Geometry check sheet. Reference: the model listing, model coordinates, mm. A direction names the side the tool comes from. Give positions to 0.01 mm unless a question says otherwise; leave off trailing zeros. Order: outer loops, then holes, each group sorted by start corner. A loop starts at its lowest first (then second) coordinate and runs counter-clockwise, first axis right, second up. Notation, with made-up numbers: (44, -32) - (55, -32) arc R16 cw to (55, -5) - close; hole circle Ø8 at (-2, 7). An arc over 180 degrees is marked (long way). Put each result on its own line as item: value. Start each with the question number.
```python
from build123d import *

# Parameters (mm, degrees)
F0_R     = 4
F0_R_2   = 1.5
F1_DEPTH = 20
F3_R     = 1.1
F4_DEPTH = 16.001


with BuildPart() as f1:
    # F0 (on Top) → F1 (new body)
    with BuildSketch(Plane.XY):
        with BuildLine():
            ThreePointArc((-8, 0), (0, -8), (8, 0))
            Line((8, 0), (8, 24))
            ThreePointArc((8, 24), (7.12132, 26.12132), (5, 27))
            Line((5, 27), (-5, 27))
            ThreePointArc((-5, 27), (-7.12132, 26.12132), (-8, 24))
            Line((-8, 24), (-8, 0))
        make_face()
        Circle(F0_R, mode=Mode.SUBTRACT)
        with Locations((-3.675823, 22.163428)):
            Circle(F0_R_2, mode=Mode.SUBTRACT)
        with Locations((3.675823, 22.163428)):
            Circle(F0_R_2, mode=Mode.SUBTRACT)
    extrude(amount=F1_DEPTH)

    # F3 (on face) → F4 (cut, through all)
    with BuildSketch(Plane(origin=(-8, 0, 0), x_dir=(0, -1, 0), z_dir=(-1, 0, 0))):
        with BuildLine():
            Line((15.480949, 34.118096), (-11.102321, 34.118096))
            Line((-11.102321, 34.118096), (-11.102321, 15))
            ThreePointArc((-11.102321, 15), (-9.637855, 11.464466), (-6.102321, 10))
            Line((-6.102321, 10), (15.473341, 10))
            Line((15.473341, 10), (15.480949, 34.118096))
        make_face()
        with BuildLine():
            Line((-19.958727, 15), (-48.31529, 15))
            Line((-48.31529, 15), (-48.31529, 0))
            Line((-48.31529, 0), (-48.31529, -8.176547))
            Line((-48.31529, -8.176547), (-5.153973, -8.176547))
            Line((-5.153973, -8.176547), (-5.153973, 0))
            ThreePointArc((-5.153973, 0), (-7.286992, 0.559089), (-9.138177, 1.757198))
            Line((-9.138177, 1.757198), (-15.357077, 7.361316))
            ThreePointArc((-15.357077, 7.361316), (-17.07554, 10.143206), (-17.97924, 13.285714))
            ThreePointArc((-17.97924, 13.285714), (-18.64942, 14.511858), (-19.958727, 15))
        make_face()
        with Locations((0, 5)):
            Circle(F3_R)
    extrude(amount=-F4_DEPTH, mode=Mode.SUBTRACT)


solid = f1.part
```
Item 1: Cross-section at A-A (x = 0). Enter the section's corners in (y, z).
Item 2: Cross-section at B-B (x = -4.5). Enter the section's corners in (y, z), and give its area (3 significant figures).
Item 3: Gauge pin test, flat ends, axial feed: pin 1 Ø6 at (x, y) = (-1.5, 1) entering from +Z; pin 2 Ø3.5 at (x, y) = (3, 23) entering from -Z; pin 3 Ø4 at (x, z) = (1.5, 17) entering from -Y. Record the tip position at first contact, or that the pin passes through.
Item 4: Cross-section at D-D (x = 3). Enter the section's corners in (y, z).
Item 5: Set-up check for faces 4 (the face through (0, 11.102, 18)), 5 (the face through (-0.1, -4.3, 0)), 6 (the face through (0, 23, 15)): record each of +Z, -Z, +X, -X, +Y, -Y from which the full face is reachable in a straight line by a thin tool's end or side.
Item 6: Cross-section at C-C (z = 2.5). Enter the section's corners in (x, y), and give its area (3 significant figures).
Item 7: Release check for a two-part mould opening along Z. For faces 1 (the face through (3.4, -2.4, 10)), 2 (the face through (-5.95, -0.59, 5.93)), 3 (the face through (-0.112, 17.057, 10.101)) record: +Z half, -Z half, draft (parallel to the pull), parting line (faces both ways), or undercut.
Item 8: Thickness scan on line 1 along Z through (x, y) = (5.5, 0); line 2 along Y through (x, z) = (1.25, 2.25); line 3 along Z through (x, y) = (-1, -5.5). Record the ranges inside material, lowest first.
Recorded:
1. outline: (-8, 0) - (-4, 0) - (-4, 10) - (-8, 10) - close; (4, 0) - (5.15, 0) arc R6.96 ccw to (9.14, 1.76) - (15.36, 7.36) arc R12 ccw to (17.98, 13.29) arc R2 cw to (19.96, 15) - (27, 15) - (27, 20) - (11.1, 20) - (11.1, 15) arc R5 cw to (6.1, 10) - (4, 10) - close
2. outline: (-6.61, 0) - (5.15, 0) arc R6.96 ccw to (9.14, 1.76) - (15.36, 7.36) arc R12 ccw to (17.98, 13.29) arc R2 cw to (19.96, 15) - (20.91, 15) - (20.91, 20) - (11.1, 20) - (11.1, 15) arc R5 cw to (6.1, 10) - (-6.61, 10) - close; (23.42, 15) - (27, 15) - (27, 20) - (23.42, 20) - close; hole circle Ø2.2 at (0, 5)
2. area: 294 mm^2
3. pin 1: stops at z = 10
3. pin 2: stops at z = 15
3. pin 3: stops at y = 11.1
4. outline: (-7.42, 0) - (-2.65, 0) - (-2.65, 10) - (-7.42, 10) - close; (2.65, 0) - (5.15, 0) arc R6.96 ccw to (9.14, 1.76) - (15.36, 7.36) arc R12 ccw to (17.98, 13.29) arc R2 cw to (19.96, 15) - (20.82, 15) - (20.82, 20) - (11.1, 20) - (11.1, 15) arc R5 cw to (6.1, 10) - (2.65, 10) - close; (23.5, 15) - (27, 15) - (27, 20) - (23.5, 20) - close
5. face 4: +Z, +X, -X, -Y
5. face 5: -Z, +X, -X, +Y, -Y
5. face 6: -Z, +X, -X, +Y
6. outline: (-8, 0) arc R8 ccw to (8, 0) - (8, 9.96) - (-8, 9.96) - close; hole circle Ø8 at (0, 0)
6. area: 210 mm^2
7. face 1: +Z half
7. face 2: undercut
7. face 3: -Z half
8. line 1: z = 0 to 3.9, 6.1 to 10
8. line 2: y = -7.9 to -3.8, 3.8 to 9.69
8. line 3: z = 0 to 10
